from build123d import *

# Parameters (mm, degrees)
ESQUISSE1_R             = 2.5
BASE_EXTRUSION_DEPTH    = 1.5
BASE_EXTRUSION_TAPER    = 8
CONG_1_R                = 0.75
CONG_2_R                = 0.25
ESQUISSE2_R             = 1.5
BOSS_EXTRU_1_DEPTH      = 27
CHANFREIN1_SIZE         = 0.5
ENL_V_MAT_EXTRU_1_DEPTH = 1
ESQUISSE5_W             = 0.5
ESQUISSE5_H             = 5.000243794
ENL_V_MAT_EXTRU_2_DEPTH = 0.75


with BuildPart() as part:
    # Esquisse1 → Base-Extrusion (new body)
    with BuildSketch(Plane.XY):
        Circle(ESQUISSE1_R)
    extrude(amount=BASE_EXTRUSION_DEPTH, taper=BASE_EXTRUSION_TAPER)

    # Congé1
    cong_1_edges = [part.edges().sort_by_distance(p)[0] for p in [
        (-2.289188748, 0, 1.5),
    ]]
    fillet(cong_1_edges, radius=CONG_1_R)

    # Congé2
    cong_2_edges = [part.edges().sort_by_distance(p)[0] for p in [
        (-2.5, 0, 0),
    ]]
    fillet(cong_2_edges, radius=CONG_2_R)

    # Esquisse2 → Boss.-Extru.1 (add)
    with BuildSketch(Plane(origin=(0, 0, 0), x_dir=(-1, 0, 0), z_dir=(0, 0, -1))):
        Circle(ESQUISSE2_R)
    extrude(amount=BOSS_EXTRU_1_DEPTH)

    # Chanfrein1
    chanfrein1_edges = [part.edges().sort_by_distance(p)[0] for p in [
        (1.5, 0, -27),
    ]]
    chamfer(chanfrein1_edges, length=CHANFREIN1_SIZE)

    # Esquisse4 → Enlèv. mat.-Extru.1 (cut)
    with BuildSketch(Plane.XY.offset(1.5)):
        with BuildLine():
            Line((-0.25, 1.75), (-0.25, 0.572821962))
            ThreePointArc((-0.25, 0.572821962), (-0.441941738, 0.441941738), (-0.572821962, 0.25))
            Line((-0.572821962, 0.25), (-1.75, 0.25))
            Line((-1.75, 0.25), (-1.75, -0.25))
            Line((-1.75, -0.25), (-0.572821962, -0.25))
            ThreePointArc((-0.572821962, -0.25), (-0.441941738, -0.441941738), (-0.25, -0.572821962))
            Line((-0.25, -0.572821962), (-0.25, -1.75))
            Line((-0.25, -1.75), (0.25, -1.75))
            Line((0.25, -1.75), (0.25, -0.572821962))
            ThreePointArc((0.25, -0.572821962), (0.441941738, -0.441941738), (0.572821962, -0.25))
            Line((0.572821962, -0.25), (1.75, -0.25))
            Line((1.75, -0.25), (1.75, 0.25))
            Line((1.75, 0.25), (0.572821962, 0.25))
            ThreePointArc((0.572821962, 0.25), (0.441941738, 0.441941738), (0.25, 0.572821962))
            Line((0.25, 0.572821962), (0.25, 1.75))
            Line((0.25, 1.75), (-0.25, 1.75))
        make_face()
    extrude(amount=-ENL_V_MAT_EXTRU_1_DEPTH, mode=Mode.SUBTRACT)

    # Esquisse5 → Enlèv. mat.-Extru.2 (cut)
    with BuildSketch(Plane.XY.offset(1.5)):
        with Locations((0, 0.01124212)):
            Rectangle(ESQUISSE5_W, ESQUISSE5_H)
    extrude(amount=-ENL_V_MAT_EXTRU_2_DEPTH, mode=Mode.SUBTRACT)


solid = part.part
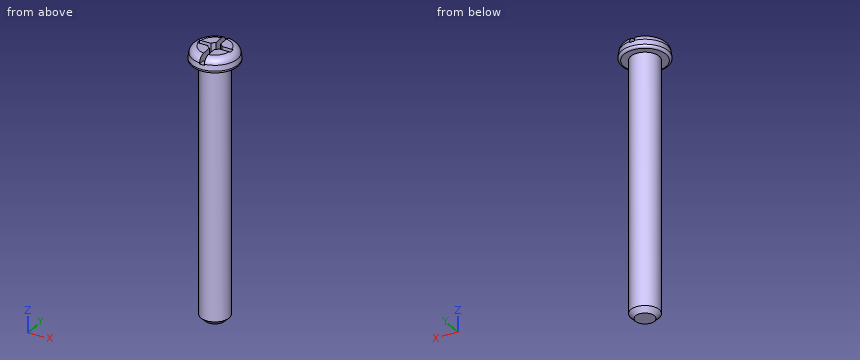
Can you work these out from the model? Positions are in its coordinate system, mm. Give positions to 0.01 mm unless a question says otherwise; leave off trailing zeros. Loops run counter-clockwise (first coordinate to the right, second up) from the corner with the lowest first, then second, coordinate; pieces in that order, holes last. Notation, with made-up numbers: (30.25, 0) - (35.25, 0) arc R28 ccw to (35.25, 29) - close; hole circle Ø2 at (21.25, 10). An arc over 180 degrees is marked (long way). One line per item, written item: value.
(1) I'm going to push flat-ended pins straight in: pin 1 (1.1 mm diameter, centred on x = -1, z = 1, fed in from -Y); pin 2 (0.5 mm diameter, centred on y = -1.5, z = 1, fed in from -X); pin 3 (1.1 mm diameter, centred on x = -1, z = 1, fed in from +Y). Where does each tip first touch, or does it pass through?
Verdict:
pin 1: y = -2.34
pin 2: x = -2
pin 3: y = 2.34
(2) If we section it at C-C, the plane z = -7: List the corners of the cut face in (x, y) for me.
Verdict:
outline: circle Ø3 at (0, 0)
(3) If we section it at A-A, the plane y = 0: List the corners of the cut face in (x, z) for me.
Verdict:
outline: (-2.46, 0.28) arc R0.25 ccw to (-2.21, 0) - (-1.5, 0) - (-1.5, -26.5) - (-1, -27) - (1, -27) - (1.5, -26.5) - (1.5, 0) - (2.21, 0) arc R0.25 ccw to (2.46, 0.28) - (2.38, 0.85) arc R0.75 ccw to (1.75, 1.49) - (1.75, 0.5) - (-1.75, 0.5) - (-1.75, 1.49) arc R0.75 ccw to (-2.38, 0.85) - close
(4) If we section it at B-B, the plane x = 0: List the corners of the cut face in (y, z) for me, plus the area to 3 significant figures.
Verdict:
outline: (-2.46, 0.28) arc R0.25 ccw to (-2.21, 0) - (-1.5, 0) - (-1.5, -26.5) - (-1, -27) - (1, -27) - (1.5, -26.5) - (1.5, 0) - (2.21, 0) arc R0.25 ccw to (2.46, 0.28) - (2.39, 0.75) - (1.75, 0.75) - (1.75, 0.5) - (-1.75, 0.5) - (-1.75, 0.75) - (-2.39, 0.75) - close
area: 83.5 mm^2
(5) I need wall thicknesses on line 1 along Y through (x, z) = (-0.05, -5); line 2 along Z through (x, y) = (-0.1, 1.55); line 3 along Z through (x, y) = (-0.75, -1.55). Which ranges of each line are inside material? Lowest first, please.
Verdict:
line 1: -1.5 to 1.5
line 2: 0 to 0.5
line 3: 0 to 1.5
